```python
from build123d import *

# Parameters (mm, degrees)
SKETCH1_R           = 2
BOSS_EXTRUDE1_DEPTH = 5
FILLET1_R           = 5
FILLET2_R           = 5
SKETCH3_R           = 3.5
CUT_EXTRUDE2_DEPTH  = 2
CIRPATTERN1_COUNT   = 2
CIRPATTERN1_ANGLE   = 90


with BuildPart() as part:
    # Sketch1 → Boss-Extrude1 (new body)
    with BuildSketch(Plane(origin=(0, 0, 0), x_dir=(1, 0, 0), z_dir=(0, 1, 0))):
        with BuildLine():
            Line((-22.5, 5), (-22.5, -5))
            Line((-22.5, -5), (-12.539936204, -5))
            ThreePointArc((-12.539936204, -5), (0, -13.5), (12.539936204, -5))
            Line((12.539936204, -5), (22.5, -5))
            Line((22.5, -5), (22.5, 5))
            Line((22.5, 5), (12.539936204, 5))
            ThreePointArc((12.539936204, 5), (0, 13.5), (-12.539936204, 5))
            Line((-12.539936204, 5), (-22.5, 5))
        make_face()
        with Locations(Location((15, 0, 0), (0, 0, 270))):
            Circle(SKETCH1_R, mode=Mode.SUBTRACT)
        with Locations(Location((-15, 0, 0), (0, 0, 270))):
            Circle(SKETCH1_R, mode=Mode.SUBTRACT)
        with Locations(Location((-7.1, 0, 0), (0, 0, 270))):
            Circle(SKETCH1_R, mode=Mode.SUBTRACT)
        with Locations(Location((7.1, 0, 0), (0, 0, 270))):
            Circle(SKETCH1_R, mode=Mode.SUBTRACT)
        with Locations(Location((0, -7.1, 0), (0, 0, 270))):
            Circle(SKETCH1_R, mode=Mode.SUBTRACT)
        with Locations(Location((0, 7.1, 0), (0, 0, 270))):
            Circle(SKETCH1_R, mode=Mode.SUBTRACT)
    extrude(amount=BOSS_EXTRUDE1_DEPTH)

    # Fillet1
    fillet1_edges = [part.edges().sort_by_distance(p)[0] for p in [
        (-22.5, 2.5, -5),
        (-22.5, 2.5, 5),
        (22.5, 2.5, 5),
        (22.5, 2.5, -5),
    ]]
    fillet(fillet1_edges, radius=FILLET1_R - 0.0001)  # a hair under: the kernel refuses the full size

    # Fillet2
    fillet2_edges = [part.edges().sort_by_distance(p)[0] for p in [
        (-12.539936204, 2.5, -5),
        (12.539936204, 2.5, -5),
        (12.539936204, 2.5, 5),
        (-12.539936204, 2.5, 5),
    ]]
    fillet(fillet2_edges, radius=FILLET2_R)

    # Sketch3 → Cut-Extrude2 (cut)
    with BuildSketch(Plane.XZ):
        with Locations(Location((-7.1, 0, 0), (0, 0, 270))):
            Circle(SKETCH3_R)
        with Locations(Location((7.1, 0, 0), (0, 0, 270))):
            Circle(SKETCH3_R)
    cut_extrude2 = extrude(amount=-CUT_EXTRUDE2_DEPTH, mode=Mode.SUBTRACT)

    # CirPattern1: Cut-Extrude2 ×2 about axis
    cirpattern1_axis = Axis((0, 0, 0), (0, 1, 0))
    for i in range(1, CIRPATTERN1_COUNT):
        add(cut_extrude2.rotate(cirpattern1_axis, i * CIRPATTERN1_ANGLE / (CIRPATTERN1_COUNT - 1)), mode=Mode.SUBTRACT)


solid = part.part
```
Source: CAD feature listing. Evaluate the final solid. Frame: model axes, mm. A direction names the side the tool comes from. Round coordinates to 2 decimals unless told otherwise and drop trailing zeros. Loops run counter-clockwise (first coordinate to the right, second up) from the corner with the lowest first, then second, coordinate; pieces in that order, holes last. Notation, with made-up numbers: M 36,49 L 77,49 A19 ccw 77,56 Z; hole C 73.5,29.5 d1. An arc over 180 degrees is marked long. Use a Markdown table: item, result. Add a question column.
1. Contact query for flat-ended pins moving along their axis: P1, Ø2, axis at x = 17, y = 2, coming from the -Z side; P2, Ø1.5, axis at y = 3.5, z = -4, coming from the +X side; P3, Ø6.5, axis at x = 0, z = -7.1, coming from the -Y side. Output: stop coordinate, or through.
2. Line query: line 1 (Z direction, x = 0, y = 3.05); line 2 (X direction, y = 3.85, z = 0); line 3 (X direction, y = 1.45, z = 0). Output: solid intervals per line, ascending.
3. Reachability of faces 1 (the flat face through (17, 2, -5)), 2 (the flat face through (17, 2, 5)), 3 (the cylindrical face through (-5.117, 3.479, -0.26)), 4 (the flat face through (-9, 2, -2)) from +Z, -Z, +X, -X, +Y, -Y: full face, straight path, thin tool, end or side. Return the list, or none.
4. Section query A-A on y = 3.4. Give the number of separate pieces and of enclosed holes in the cut face, then the cut area to 3 significant figures.
5. Section query D-D on z = 8.25. Return the cut outline in (x, y), then the cut area to 3 significant figures.
6. Section query C-C on x = 14. Return the cut outline in (y, z).
7. Section query B-B on x = 0. Return the cut outline in (y, z).
8. Mould query, pull axis Z, two halves, no side actions, for faces 5 (the cylindrical face through (-21.07, 2.54, -3.5)), 6 (the cylindrical face through (-0.2, 2.5, 13.5)), 7 (the cylindrical face through (-0.766, 3.479, 8.947)). Classes: pulls with the +Z half, pulls with the -Z half, needs draft (parallel to the pull), parting line crosses it, or undercut.
Reported:
| question | item | result |
|---|---|---|
| 1 | P1 | stops at z = -5 |
| 1 | P2 | stops at x = 21.3 |
| 1 | P3 | stops at y = 2 |
| 2 | line 1 | z = -13.5 to -9.1, -5.1 to 5.1, 9.1 to 13.5 |
| 2 | line 2 | x = -22.5 to -17, -13 to -9.1, -5.1 to 5.1, 9.1 to 13, 17 to 22.5 |
| 2 | line 3 | x = -22.5 to -17, -13 to -10.6, -3.6 to 3.6, 10.6 to 13, 17 to 22.5 |
| 3 | face 1 | -Z, +X, +Y, -Y |
| 3 | face 2 | +Z, +X, +Y, -Y |
| 3 | face 3 | +Y, -Y |
| 3 | face 4 | -Y |
| 4 | separate pieces | 1 |
| 4 | enclosed holes | 6 |
| 4 | area | 668 mm² |
| 5 | outline | M -10.69,0 L -3.31,0 L -3.31,2 L -1.64,2 L -1.64,5 L -10.69,5 Z; M 1.64,2 L 3.31,2 L 3.31,0 L 10.69,0 L 10.69,5 L 1.64,5 Z |
| 5 | area | 83.8 mm² |
| 6 | outline | M 0,-5.25 L 5,-5.25 L 5,-1.73 L 0,-1.73 Z; M 0,1.73 L 5,1.73 L 5,5.25 L 0,5.25 Z |
| 7 | outline | M 0,-13.5 L 5,-13.5 L 5,-9.1 L 2,-9.1 L 2,-10.6 L 0,-10.6 Z; M 0,-3.6 L 2,-3.6 L 2,-5.1 L 5,-5.1 L 5,5.1 L 2,5.1 L 2,3.6 L 0,3.6 Z; M 0,10.6 L 2,10.6 L 2,9.1 L 5,9.1 L 5,13.5 L 0,13.5 Z |
| 8 | face 5 | pulls with the -Z half |
| 8 | face 6 | pulls with the +Z half |
| 8 | face 7 | undercut |
